Work out the finished part from the listing and answer in its coordinate system (mm). A direction names the side the tool comes from. Give positions to 0.01 mm unless a question says otherwise; leave off trailing zeros. Loops run counter-clockwise (first coordinate to the right, second up) from the corner with the lowest first, then second, coordinate; pieces in that order, holes last. Notation, with made-up numbers: M -13.75,89 L 43.25,89 A8 cw 43.25,100 Z; hole C -17,57 d5. An arc over 180 degrees is marked long. Answer as a JSON object with one key per item and string values. Group by question number.
```python
from build123d import *

# Parameters (mm, degrees)
F1_DEPTH = 12.7
F2_R     = 41.91
F3_DEPTH = 6.35
F5_DEPTH = 6.35
F5_TAPER = -10


with BuildPart() as f1:
    # F0 (on Top) → F1 (new body)
    with BuildSketch(Plane.XY):
        with BuildLine():
            Line((-21.2985474857, 6.35), (-47.8404128327, 6.35))
            ThreePointArc((-47.8404128327, 6.35), (-48.26, 0), (-47.8404128327, -6.35))
            Line((-47.8404128327, -6.35), (-21.2985474857, -6.35))
            ThreePointArc((-21.2985474857, -6.35), (-22.225, 0), (-21.2985474857, 6.35))
        make_face()
        with BuildLine():
            ThreePointArc((22.225, 0), (21.9921672746, 3.2086139633), (21.2985474857, 6.35))
            Line((21.2985474857, 6.35), (-21.2985474857, 6.35))
            ThreePointArc((-21.2985474857, 6.35), (-22.225, 0), (-21.2985474857, -6.35))
            Line((-21.2985474857, -6.35), (21.2985474857, -6.35))
            ThreePointArc((21.2985474857, -6.35), (21.9921672746, -3.2086139633), (22.225, 0))
        make_face()
        with BuildLine():
            ThreePointArc((47.8404128327, -6.35), (48.1549889591, -3.1819236867), (48.26, 0))
            ThreePointArc((48.26, 0), (48.1549889591, 3.1819236867), (47.8404128327, 6.35))
            Line((47.8404128327, 6.35), (21.2985474857, 6.35))
            ThreePointArc((21.2985474857, 6.35), (21.9921672746, 3.2086139633), (22.225, 0))
            ThreePointArc((22.225, 0), (21.9921672746, -3.2086139633), (21.2985474857, -6.35))
            Line((21.2985474857, -6.35), (47.8404128327, -6.35))
        make_face()
        with BuildLine():
            ThreePointArc((-21.2985474857, -6.35), (0, -22.225), (21.2985474857, -6.35))
            Line((21.2985474857, -6.35), (-21.2985474857, -6.35))
        make_face()
        with BuildLine():
            Line((-21.2985474857, 6.35), (21.2985474857, 6.35))
            ThreePointArc((21.2985474857, 6.35), (0, 22.225), (-21.2985474857, 6.35))
        make_face()
    extrude(amount=F1_DEPTH)

    # F2 (on face) → F3 (cut)
    with BuildSketch(Plane.XY.offset(12.7)):
        Circle(F2_R)
    extrude(amount=-F3_DEPTH, mode=Mode.SUBTRACT)

    # F4 (on face) → F5 (cut, through all)
    with BuildSketch(Plane.XY.offset(6.35)):
        with BuildLine():
            ThreePointArc((-16.51, 0), (0, 16.51), (16.51, 0))
            Line((16.51, 0), (16.51, 14.8785256326))
            ThreePointArc((16.51, 14.8785256326), (0, 22.225), (-16.51, 14.8785256326))
            Line((-16.51, 14.8785256326), (-16.51, 0))
        make_face()
        with BuildLine():
            ThreePointArc((-16.51, 0), (0, -16.51), (16.51, 0))
            ThreePointArc((16.51, 0), (0, 16.51), (-16.51, 0))
        make_face()
    extrude(amount=-F5_DEPTH, taper=F5_TAPER, mode=Mode.SUBTRACT)


solid = f1.part
```
Item 1: Given pin 1 Ø12 at (x, y) = (12, -2.5) entering from +Z; pin 2 Ø6.5 at (x, z) = (39.5, 4.5) entering from +Y; pin 3 Ø4 at (y, z) = (6, 11) entering from +X, each flat-ended and moving along its own axis, determine where each tip first touches the part or whether it passes through.
Item 2: A tool of negligible diameter and unlimited length cuts with its end or side. For faces 4 (the flat face through (37, -6.35, 5)), 5 (the cylindrical face through (-41.91, 0.09, 9.57)), 6 (the flat face through (-37, 6.35, 5)), from which of +Z, -Z, +X, -X, +Y, -Y can it reach the whole face along a straight path? Write none if from no direction.
Item 3: For a pull along Y with two mould halves and no side action, classify faces 1 (the cylindrical face through (-48.26, 0.09, 6.26)), 2 (the cylindrical face through (41.91, -0.09, 9.57)), 3 (the flat face through (45, 0, 12.7)) as pulls with the +Y half, pulls with the -Y half, needs draft (parallel to the pull), parting line crosses it, or undercut.
Item 4: Find the intervals of material crossed by probe 1 along Y at (x, z) = (31, 4.25); probe 2 along Z at (x, y) = (15.5, -14); probe 3 along X at (y, z) = (4.5, 9.5), in increasing order. Write a range as [from, to].
Item 5: A cutting plane is placed at B-B (y = -20). Determine the outline of the cut face in (x, z).
Item 6: A cutting plane is placed at A-A (x = -40). Determine the outline of the cut face in (y, z), and give its area (3 significant figures).
The answers:
{
 "1": {"pin 1": "stops at z = 6.35", "pin 2": "stops at y = 6.35", "pin 3": "stops at x = 48.09"},
 "2": {"face 4": "+Z, -Z, +X, -Y", "face 5": "+Z", "face 6": "+Z, -Z, -X, +Y"},
 "3": {"face 1": "parting line crosses it", "face 2": "undercut", "face 3": "needs draft"},
 "4": {"probe 1": "y = [-6.35, 6.35]", "probe 2": "z = [0, 6.35]", "probe 3": "x = [-48.05, -41.67], [41.67, 48.05]"},
 "5": {"outline": "M -9.69,0 L 9.69,0 L 9.69,6.35 L -9.69,6.35 Z"},
 "6": {"outline": "M -6.35,0 L 6.35,0 L 6.35,6.35 L -6.35,6.35 Z", "area": "80.6 mm^2"}
}
